The model under review builds one solid part; all positions refer to its coordinate system, in mm. Face numbers are marked on the shaded views. Give positions to 0.01 mm unless a question says otherwise; leave off trailing zeros. Write each loop counter-clockwise with the first axis right and the second up, starting at its lowest first coordinate (ties: lowest second). Pieces come first, ordered by that corner, then holes. Notation, with made-up numbers: (6, -7.75) - (27, -7.75) arc R6 ccw to (27, -3.75) - close; hole circle Ø3 at (4.5, -8.75). An arc over 180 degrees is marked (long way). One line per question, with ' | ' between items. Start each with the question number.
Autodesk Inventor part; units mm, degrees
ref_plane "YZ Plane" through (0, 0, 0) normal (1, 0, 0) x (0, 1, 0)
ref_plane "XZ Plane" through (0, 0, 0) normal (0, 1, 0) x (-1, 0, 0)
ref_plane "XY Plane" through (0, 0, 0) normal (0, 0, 1) x (1, 0, 0)
sketch "Sketch1" plane through (0, 0, 0) normal (0, 1, 0) x (-1, 0, 0)
  circle A0 centre (0, 0) radius 10 construction
  circle A1 centre (0, 0) radius 23.5
  circle A2 centre (0, 0) radius 100
  circle A3 centre (0, 0) radius 18.5
  dimension "d0" = 20
  dimension "d1" = 47
  dimension "d2" = 200
  dimension "d3" = 37
extrude "Extrusion1" add sketch "Sketch1" along normal blind 30 contours A2
extrude "Extrusion2" add sketch "Sketch1" along normal blind 15 contours A1
sketch "Sketch2" plane through (0, 0, 0) normal (0, -1, 0) x (1, 0, 0)
  circle A0 centre (0, 0) radius 25 construction
  circle A1 centre (0, -50) radius 25 construction
  circle A2 centre (0, 0) radius 31
  circle A3 centre (0, -50) radius 31
  dimension "dp" = 50
  dimension "d9" = 50
  dimension "d10" = 62
  dimension "d11" = 62
extrude "Extrusion3" cut sketch "Sketch2" against normal blind 10 contours A2 A3 | A3 A2 picked at (0.2237, 14.1835) picked at (-2.1631, -26.7711)
extrude "Extrusion4" cut sketch "Sketch2" against normal blind 10 contours A3 A2 | A2 A3 picked at (-2.1631, -26.7711) picked at (0.2237, -64.1835)
pattern_circular "Circular Pattern1" count 5 over 360 about axis through (0, 0, 0) along (0, 1, 0) of "Extrusion4"
equation "\"d9\" = dp"
equation "\"d11\" = d10"
equation "\"d14\" = d12"
equation "\"modul\" = 2"
properties part number "TERMINAL-GEAR-BASE"
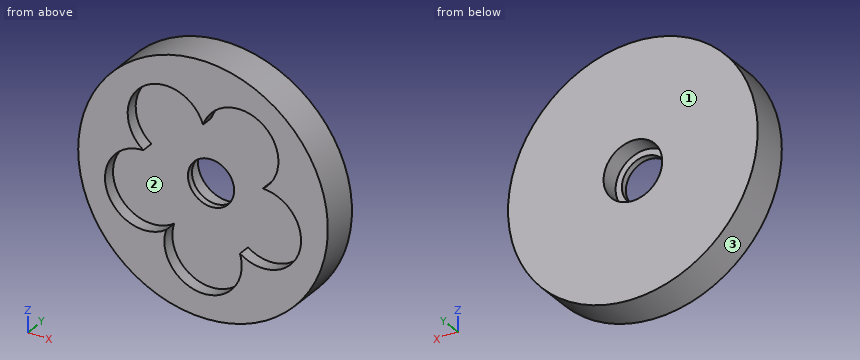
Item 1: Clearance check with flat-ended pins moving along their axes: P1, Ø8, axis at y = 10.5, z = -25, coming from the +X side; P2, Ø10, axis at x = 27, y = 15, coming from the -Z side; P3, Ø6, axis at x = 41.5, z = -69.5, coming from the -Y side; P4, Ø10, axis at y = 10, z = -49.5, coming from the -X side. State where each tip first meets the part, or that it passes through.
Item 2: Take a section at A-A (x = -9). Give the boundary of the cut face in (y, z).
Item 3: Take a section at D-D (z = -30.5). Give the boundary of the cut face in (x, y).
Item 4: Take a section at B-B (z = 0). Give the boundary of the cut face in (x, y), plus the area to 3 significant figures.
Item 5: For probe 1 along Z at (x, y) = (0, 12.2); probe 2 along Y at (x, z) = (28.5, -3.5); probe 3 along Z at (x, y) = (0, 21.75), list the stretches that pass through material, from the lowest coordinate up.
Item 6: The part is to be moulded in two halves that separate along X. For the marked faces 1, 2 and 3, say which applies: +X half, -X half, draft (parallel to the pull), parting line (faces both ways), or undercut.
Item 7: Take a section at C-C (y = 26.5). Give the boundary of the cut face in (x, z), plus the area to 3 significant figures.
Check sheet entries:
1) P1: stops at x = 97.77 | P2: stops at z = -97.55 | P3: stops at y = 0 | P4: stops at x = -89.55
2) outline: (0, -99.59) - (30, -99.59) - (30, -21.71) - (15, -21.71) - (15, -16.16) - (10, -16.16) - (10, -79.66) - (0, -79.66) - close; (0, 63.8) - (10, 63.8) - (10, 16.16) - (15, 16.16) - (15, 21.71) - (30, 21.71) - (30, 99.59) - (0, 99.59) - close
3) outline: (-95.24, 0) - (-74.65, 0) - (-74.65, 10) - (74.65, 10) - (74.65, 0) - (95.24, 0) - (95.24, 30) - (-95.24, 30) - close
4) outline: (-100, 0) - (-74.43, 0) - (-74.43, 10) - (-18.5, 10) - (-18.5, 15) - (-23.5, 15) - (-23.5, 30) - (-100, 30) - close; (18.5, 10) - (74.43, 10) - (74.43, 0) - (100, 0) - (100, 30) - (23.5, 30) - (23.5, 15) - (18.5, 15) - close | area: 3,620 mm^2
5) probe 1: z = -100 to -18.5, 18.5 to 100 | probe 2: y = 10 to 30 | probe 3: z = -100 to -23.5, 23.5 to 100
6) face 1: draft | face 2: undercut | face 3: parting line
7) outline: circle Ø200 at (0, 0); hole circle Ø47 at (0, 0) | area: 29,700 mm^2
